```python
from build123d import *

# Parameters (mm, degrees)
F0_W     = 25.4
F0_H     = 31.75
F1_DEPTH = 38.1
F2_W     = 12.7
F2_H     = 19.05
F3_DEPTH = 38.1
F5_DEPTH = 25.4
F7_DEPTH = 25.4


with BuildPart() as f1:
    # F0 (on Front) → F1 (new body)
    with BuildSketch(Plane.XZ):
        with Locations((-12.7, 15.875)):
            Rectangle(F0_W, F0_H)
    extrude(amount=F1_DEPTH)

    # F2 (on face) → F3 (cut)
    with BuildSketch(Plane.XZ.offset(38.1)):
        with Locations((-19.05, 22.225)):
            Rectangle(F2_W, F2_H)
    extrude(amount=-F3_DEPTH, mode=Mode.SUBTRACT)

    # F4 (on face) → F5 (cut)
    with BuildSketch(Plane.XY.offset(12.7)):
        Polygon((-25.4, -38.1), (-12.7, -38.1), (-25.4, -25.3298), align=None)
    extrude(amount=-F5_DEPTH, mode=Mode.SUBTRACT)

    # F6 (on face) → F7 (cut)
    with BuildSketch(Plane(origin=(-12.7, 0, 0), x_dir=(0, -1, 0), z_dir=(-1, 0, 0))):
        Polygon((24.324648, 31.75), (38.1, 12.7), (38.1, 31.75), align=None)
    extrude(amount=-F7_DEPTH, mode=Mode.SUBTRACT)


solid = f1.part
```
Verification items for the finished model (mm, model axes). A direction names the side the tool comes from. Round coordinates to 2 decimals unless told otherwise and drop trailing zeros. Order: outer loops, then holes, each group sorted by start corner. A loop starts at its lowest first (then second) coordinate and runs counter-clockwise, first axis right, second up.
1) Cross-section at A-A, the plane z = 6. Record the cut outline in (x, y), plus the area to 3 significant figures.
Geometry says:
outline: (-25.4, -25.33) - (-12.7, -38.1) - (0, -38.1) - (0, 0) - (-25.4, 0) - close
area: 887 mm2
2) Tool access check on faces 1 (the flat face through (-19, -15, 12.7)), 2 (the flat face through (-10, 0, 13)). Record the directions out of +Z, -Z, +X, -X, +Y, -Y that give a thin tool (end or side, any length) a straight path to the whole face; none if there is none.
Geometry says:
face 1: +Z, -X, +Y, -Y
face 2: +Z, -Z, +X, -X, +Y
3) Cross-section at C-C, the plane x = -5.75. Record the cut outline in (y, z).
Geometry says:
outline: (-38.1, 0) - (0, 0) - (0, 31.75) - (-24.32, 31.75) - (-38.1, 12.7) - close
4) Material ranges on line 1 (X direction, y = -11, z = 26); line 2 (Z direction, x = -17, y = -14.5); line 3 (Y direction, x = -9, z = 13), recorded low to high.
Geometry says:
line 1: x = -12.7 to 0
line 2: z = 0 to 12.7
line 3: y = -37.88 to 0
5) Depth check by flat-ended pin: pin 1 (12 mm diameter, centred on x = -10.5, z = 25.5, fed in from -Y); pin 2 (12 mm diameter, centred on x = -22, y = -18, fed in from +Z); pin 3 (9.5 mm diameter, centred on y = -12, z = 20.5, fed in from -X). Enter the tip coordinate at first touch or a pass-through.
Geometry says:
pin 1: stops at y = -33.18
pin 2: stops at z = 12.7
pin 3: stops at x = -12.7
6) Cross-section at D-D, the plane y = -34. Record the cut outline in (x, z).
Geometry says:
outline: (-16.78, 0) - (0, 0) - (0, 18.37) - (-12.7, 18.37) - (-12.7, 12.7) - (-16.78, 12.7) - close
7) Cross-section at B-B, the plane y = -9. Record the cut outline in (x, z), plus the area to 3 significant figures.
Geometry says:
outline: (-25.4, 0) - (0, 0) - (0, 31.75) - (-12.7, 31.75) - (-12.7, 12.7) - (-25.4, 12.7) - close
area: 565 mm2
